Model file for the job. Use its own axes, mm. A direction names the side the tool comes from. Round coordinates to 2 decimals unless told otherwise and drop trailing zeros. Order: outer loops, then holes, each group sorted by start corner. A loop starts at its lowest first (then second) coordinate and runs counter-clockwise, first axis right, second up. Notation, with made-up numbers: (-26, 69.5) -> (-15, 69.5) arc R27 ccw to (-15, 99.5) -> close; hole circle Ø2 at (-10.75, -31). An arc over 180 degrees is marked (long way). Answer as CSV lines item,"result".
Autodesk Inventor part; units mm, degrees
ref_plane "YZ Plane" through (0, 0, 0) normal (1, 0, 0) x (0, 1, 0)
ref_plane "XZ Plane" through (0, 0, 0) normal (0, 1, 0) x (-1, 0, 0)
ref_plane "XY Plane" through (0, 0, 0) normal (0, 0, 1) x (1, 0, 0)
sketch "Sketch1" plane through (0, 0, 0) normal (0, 0, 1) x (1, 0, 0)
  line L0 (50, -12.5) -> (-50, -12.5)
  line L1 (-50, -12.5) -> (-50, 12.5)
  line L2 (-50, 12.5) -> (50, 12.5)
  line L3 (50, 12.5) -> (50, -12.5)
  line L4 (50, -12.5) -> (-50, 12.5) construction
  line L5 (-50, -12.5) -> (50, 12.5) construction
  line L6 (-10, -5) -> (-40, -5)
  line L7 (-40, -5) -> (-40, 5)
  line L8 (-40, 5) -> (-10, 5)
  line L9 (-10, 5) -> (-10, -5)
  line L10 (-10, -5) -> (-40, 5) construction
  line L11 (-40, -5) -> (-10, 5) construction
  line L12 (10.2094, -6.5) -> (40.2094, -6.5)
  line L13 (40.2094, -6.5) -> (40.2094, 6.5)
  line L14 (40.2094, 6.5) -> (10.2094, 6.5)
  line L15 (10.2094, 6.5) -> (10.2094, -6.5)
  line L16 (10.2094, -6.5) -> (40.2094, 6.5) construction
  line L17 (40.2094, -6.5) -> (10.2094, 6.5) construction
  point P0 (0, 0)
  point P1 (-40, 0)
  point P2 (40, 0)
  point P3 (-25, 0)
  point P4 (25.2094, 0)
  dimension "d0" = 100
  dimension "d1" = 25
  dimension "d2" = 10
  dimension "d3" = 13
extrude "Extrusion1" add sketch "Sketch1" along normal blind 18
sketch "M6 thru" plane through (50, -12.5, 0) normal (1, 0, 0) x (0, 0, -1)
  line L0 (0, 25) -> (0, 0)
  point P0 (0, 12.5)
  point P1 (-7, 12.5)
  dimension "d13" = 7
sketch "Sketch3" plane through (-50, -12.5, 0) normal (-1, 0, 0) x (0, 0, 1)
  line L0 (0, 0) -> (0, 25)
  point P0 (0, 12.5)
  point P1 (12, 12.5)
  dimension "d14" = 12
hole "M6 thru-hole" at (50, 0, 7) direction (-1, 0, 0) diameter 6.4 end up to surface
hole "M4 thru-hole" at (-50, 0, 12) direction (1, 0, 0) diameter 4.4 end up to surface
chamfer "Chamfer1" distance 5 angle 45 4 edges at (-10, 0, 18) (10.2094, 0, 18) (-10, 0, 0) (10.2094, 0, 0)
properties part number "cage2table-mount-M4(top)-M6(bottom)-H100mm-HoleOffset5mm"
Q1. Wall check: L1, parallel to Z at x = 43.5, y = 0; L2, parallel to Y at x = 47.5, z = 7; L3, parallel to Z at x = -48, y = 0. Give the ranges that are in metal, low to high. Write a range as [from, to].
Checks:
L1,"[0, 3.8], [10.2, 18]"
L2,"[-12.5, -3.2], [3.2, 12.5]"
L3,"[0, 9.8], [14.2, 18]"
Q2. Flat gauge pins, fed straight in: pin 1 (3.5 mm diameter, centred on y = 0, z = 12, fed in from -X); pin 2 (12 mm diameter, centred on x = -14, y = 4.5, fed in from +Z). Where does each tip first touch, or does it go through?
Checks:
pin 1,"x = -10"
pin 2,"z = 18"
Q3. Saw through at D-D (x = -7). Write the cut outline in (y, z).
Checks:
outline,"(-12.5, 0) -> (-5, 0) -> (-5, 2) -> (5, 2) -> (5, 0) -> (12.5, 0) -> (12.5, 18) -> (5, 18) -> (5, 16) -> (-5, 16) -> (-5, 18) -> (-12.5, 18) -> close"
Q4. Saw through at A-A (x = -29). Write the cut outline in (y, z).
Checks:
outline,"(-12.5, 0) -> (-5, 0) -> (-5, 18) -> (-12.5, 18) -> close; (5, 0) -> (12.5, 0) -> (12.5, 18) -> (5, 18) -> close"
Q5. Mould opens along X. For faces 1 (the flat face through (-50, 0, 9)), 2 (the flat face through (-1, 0, 18)), 3 (the flat face through (-22, -5, 9)) say: +X half, -X half, draft (parallel to the pull), parting line (faces both ways), or undercut.
Checks:
face 1,"-X half"
face 2,"draft"
face 3,"undercut"
Q6. Tool access for faces 4 (the cylindrical face through (45.036, 1.226, 4.044)), 5 (the flat face through (-10, 0, 9)), 6 (the cylindrical face through (-44.93, 0.843, 14.032)): list every direction of +Z, -Z, +X, -X, +Y, -Y with a clear straight run to the whole face (end or side of a thin tool).
Checks:
face 4,"+X"
face 5,"+Z, -Z"
face 6,"-X"
Q7. Saw through at C-C (z = 7). Write the cut outline in (x, y), plus the area to 3 significant figures.
Checks:
outline,"(-50, -12.5) -> (50, -12.5) -> (50, -3.2) -> (40.21, -3.2) -> (40.21, -6.5) -> (10.21, -6.5) -> (10.21, 6.5) -> (40.21, 6.5) -> (40.21, 3.2) -> (50, 3.2) -> (50, 12.5) -> (-50, 12.5) -> close; hole (-40, -5) -> (-10, -5) -> (-10, 5) -> (-40, 5) -> close"
area,"1,750 mm²"
Q8. Saw through at B-B (y = 0). Write the cut outline in (x, z), plus the area to 3 significant figures.
Checks:
outline,"(-50, 0) -> (-40, 0) -> (-40, 9.8) -> (-50, 9.8) -> close; (-50, 14.2) -> (-40, 14.2) -> (-40, 18) -> (-50, 18) -> close; (-10, 5) -> (-5, 0) -> (5.21, 0) -> (10.21, 5) -> (10.21, 13) -> (5.21, 18) -> (-5, 18) -> (-10, 13) -> close; (40.21, 0) -> (50, 0) -> (50, 3.8) -> (40.21, 3.8) -> close; (40.21, 10.2) -> (50, 10.2) -> (50, 18) -> (40.21, 18) -> close"
area,"563 mm²"
